Geometry check sheet. Reference: the model listing, model coordinates, mm. A direction names the side the tool comes from. Coordinates: 2 decimals unless noted, no trailing zeros. Write each loop counter-clockwise with the first axis right and the second up, starting at its lowest first coordinate (ties: lowest second). Pieces come first, ordered by that corner, then holes. Notation, with made-up numbers: (6, 34) -> (11, 34) arc R24 ccw to (11, 50) -> close; hole circle Ø5 at (50, 32.5). An arc over 180 degrees is marked (long way). Answer in a Markdown table with one row per item. Add a question column.
Q1. Section check A-A, the plane x = 4. Record the boundary of the cut face in (y, z), and give its area (3 significant figures).
Q2. Release check for a two-part mould opening along X. For faces 4 (the face through (29.15, -29.75, -31.65)), 5 (the face through (-63.363, -29, -23)), 6 (the face through (-20, -37, -12.512)), 7 (the face through (-41.681, -29.748, -31.473)) record: pulls with the +X half, pulls with the -X half, needs draft (parallel to the pull), parting line crosses it, or undercut.
Q3. Section check C-C, the plane y = -47. Record the boundary of the cut face in (x, z), and give its area (3 significant figures).
Q4. Tool access check on faces 1 (the face through (-6, -23, -25.212)), 2 (the face through (-7, -15.748, 4)), 3 (the face through (-51, -29, -37.912)). Record the directions out of +Z, -Z, +X, -X, +Y, -Y that give a thin tool (end or side, any length) a straight path to the whole face; none if there is none.
Q5. Section check D-D, the plane z = -28.5. Record the boundary of the cut face in (x, y).
Q6. Thickness scan on line 1 (Y direction, x = -55.5, z = -3); line 2 (Z direction, x = -42.5, y = -25); line 3 (X direction, y = -22, z = -29). Record the ranges inside material, lowest first.
Q7. Section check B-B, the plane z = -22. Record the boundary of the cut face in (x, y).
Q8. Gauge pin test, flat ends, axial feed: P1, Ø13, axis at x = -2, y = -44, coming from the +Z side; P2, Ø5, axis at x = 37, y = -15.5, coming from the +Z side; P3, Ø16, axis at x = 0.5, z = 8, coming from the -Y side; P4, Ø10, axis at x = -36, z = 8.5, coming from the +Y side. Record the tip position at first contact, or that the pin passes through.
```python
from build123d import *

# Parameters (mm, degrees)
F0_W     = 114.3
F0_H     = 57.15
F1_DEPTH = 58.674
F2_W     = 114.3
F2_H     = 42.926
F3_DEPTH = 31.75
F5_DEPTH = 15.748
F7_DEPTH = 58.674
F9_DEPTH = 12.7


with BuildPart() as f1:
    # F0 (on Front) → F1 (new body)
    with BuildSketch(Plane.XZ):
        with Locations((-6.213398, -9.336713)):
            Rectangle(F0_W, F0_H)
    extrude(amount=F1_DEPTH)

    # F2 (on face) → F3 (cut)
    with BuildSketch(Plane.XY.offset(19.238287)):
        with Locations((-6.213398, -37.211)):
            Rectangle(F2_W, F2_H)
    extrude(amount=-F3_DEPTH, mode=Mode.SUBTRACT)

    # F4 (on face) → F5 (cut)
    with BuildSketch(Plane.XZ.offset(15.748)):
        Polygon((50.936602, 19.238287), (31.886602, 19.238287), (50.936602, 0.188287), align=None)
        Polygon((-44.313398, 19.238287), (-63.363398, 19.238287), (-63.363398, 0.188287), align=None)
    extrude(amount=-F5_DEPTH, mode=Mode.SUBTRACT)

    # F6 (on face) → F7 (cut)
    with BuildSketch(Plane.XZ.offset(58.674)):
        Polygon((-37.963398, -37.911713), (25.536602, -37.911713), (32.86895, -25.211713), (25.536602, -25.211713), (-37.963398, -25.211713), (-45.295746, -25.211713), align=None)
    extrude(amount=-F7_DEPTH, mode=Mode.SUBTRACT)

    # F8 (on face) → F9 (cut)
    with BuildSketch(Plane.XY.offset(-12.511713)):
        with BuildLine():
            ThreePointArc((6.486602, -36.576), (-15.193654, -27.595744), (-6.213398, -49.276))
            ThreePointArc((-6.213398, -49.276), (2.766858, -45.556256), (6.486602, -36.576))
        make_face()
    extrude(amount=-F9_DEPTH, mode=Mode.SUBTRACT)


solid = f1.part
```
Calculated:
| question | item | result |
|---|---|---|
| 1 | outline | (-58.67, -25.21) -> (-44.12, -25.21) -> (-44.12, -12.51) -> (-58.67, -12.51) -> close; (-29.03, -25.21) -> (0, -25.21) -> (0, 19.24) -> (-15.75, 19.24) -> (-15.75, -12.51) -> (-29.03, -12.51) -> close |
| 1 | area | 1,050 mm² |
| 2 | face 4 | undercut |
| 2 | face 5 | pulls with the -X half |
| 2 | face 6 | needs draft |
| 2 | face 7 | undercut |
| 3 | outline | (-63.36, -37.91) -> (-37.96, -37.91) -> (-45.3, -25.21) -> (-13.47, -25.21) -> (-13.47, -12.51) -> (-63.36, -12.51) -> close; (1.04, -25.21) -> (32.87, -25.21) -> (25.54, -37.91) -> (50.94, -37.91) -> (50.94, -12.51) -> (1.04, -12.51) -> close |
| 3 | area | 1,820 mm² |
| 4 | face 1 | +Y, -Y |
| 4 | face 2 | +Z, +X, -X, -Y |
| 4 | face 3 | -Z, +X, -X, +Y, -Y |
| 5 | outline | (-63.36, -58.67) -> (-43.4, -58.67) -> (-43.4, 0) -> (-63.36, 0) -> close; (30.97, -58.67) -> (50.94, -58.67) -> (50.94, 0) -> (30.97, 0) -> close |
| 6 | line 1 | y = -15.75 to 0 |
| 6 | line 2 | z = -37.91 to -30.05, -25.21 to -12.51 |
| 6 | line 3 | x = -63.36 to -43.11, 30.68 to 50.94 |
| 7 | outline | (-63.36, -58.67) -> (50.94, -58.67) -> (50.94, 0) -> (-63.36, 0) -> close; hole circle Ø25.4 at (-6.21, -36.58) |
| 8 | P1 | stops at z = -12.51 |
| 8 | P2 | stops at z = 16.62 |
| 8 | P3 | stops at y = -15.75 |
| 8 | P4 | stops at y = 0 |
